Part model, mm, in its own coordinate system. A direction names the side the tool comes from. Round coordinates to 2 decimals unless told otherwise and drop trailing zeros. Loops run counter-clockwise (first coordinate to the right, second up) from the corner with the lowest first, then second, coordinate; pieces in that order, holes last.
from build123d import *

# Parameters (mm, degrees)
BOSS_EXTRUDE2_DEPTH                               = 5.08
CSK_FOR_8_FLAT_HEAD_MACHINE_SCREW_100_D           = 4.4958
CSK_FOR_8_FLAT_HEAD_MACHINE_SCREW_100_CSINK_D     = 8.89
CSK_FOR_8_FLAT_HEAD_MACHINE_SCREW_100_CSINK_ANGLE = 100
CUT_EXTRUDE1_DEPTH                                = 4.556
FILLET1_R                                         = 2.54
FILLET2_R                                         = 1.27


with BuildPart() as part:
    # Sketch4 → Boss-Extrude2 (new body, symmetric)
    with BuildSketch(Plane.XY):
        Polygon((0, 0), (4.445, 0), (4.445, 4.572), (8.001, 4.572), (8.001, -3.81), (0, -3.81), align=None)
    extrude(amount=BOSS_EXTRUDE2_DEPTH, both=True)

    # CSK for #8 Flat Head Machine Screw (100)2 (through all)
    with Locations(Plane(origin=(0, 0, 0), x_dir=(1, 0, 0), z_dir=(0, 1, 0))):
        with Locations((0, 0)):
            CounterSinkHole(CSK_FOR_8_FLAT_HEAD_MACHINE_SCREW_100_D / 2, CSK_FOR_8_FLAT_HEAD_MACHINE_SCREW_100_CSINK_D / 2, counter_sink_angle=CSK_FOR_8_FLAT_HEAD_MACHINE_SCREW_100_CSINK_ANGLE)

    # Sketch7 → Cut-Extrude1 (cut, through all)
    with BuildSketch(Plane.ZY.offset(-4.445)):
        with BuildLine():
            Line((-1.778, 2.032), (1.778, 2.032))
            ThreePointArc((1.778, 2.032), (2.794, 1.016), (1.778, 0))
            Line((1.778, 0), (-1.778, 0))
            ThreePointArc((-1.778, 0), (-2.794, 1.016), (-1.778, 2.032))
        make_face()
    extrude(amount=-CUT_EXTRUDE1_DEPTH, mode=Mode.SUBTRACT)

    # Fillet1
    fillet1_edges = [part.edges().sort_by_distance(p)[0] for p in [
        (6.223, 4.572, 5.08),
        (6.223, 4.572, -5.08),
    ]]
    fillet(fillet1_edges, radius=FILLET1_R)

    # Fillet2
    fillet2_edges = [part.edges().sort_by_distance(p)[0] for p in [
        (8.001, -0.889, 5.08),
        (8.001, 4.572, 0),
        (8.001, 3.828051224, 4.336051224),
        (8.001, 3.828051224, -4.336051224),
        (8.001, -0.889, -5.08),
    ]]
    fillet(fillet2_edges, radius=FILLET2_R)

    # Mirror2: part across plane


with BuildPart() as part_1:
    add(part.part)
    add(part.part.mirror(Plane(origin=(0, 0, 0), x_dir=(0, 0, 1), z_dir=(1, 0, 0))))


solid = part_1.part
1) Wall check: line 1 along Z through (x, y) = (0, -2.35); line 2 along X through (y, z) = (-2.4, 0); line 3 along Y through (x, z) = (-4.5, -1). Give the ranges that are in metal, low to high.
Values:
line 1: z = -5.08 to -2.25, 2.25 to 5.08
line 2: x = -8 to -2.25, 2.25 to 8
line 3: y = -3.81 to 0, 2.03 to 4.57
2) Slice it at D-D, the plane x = 0. Give the cut face in (y, z) (3 decimals).
Values:
outline: (-3.81, -5.08) - (0, -5.08) - (0, -4.445) - (-1.844, -2.248) - (-3.81, -2.248) - close; (-3.81, 2.248) - (-1.844, 2.248) - (0, 4.445) - (0, 5.08) - (-3.81, 5.08) - close
3) Mould opens along Y. For faces 4 (the face through (-7.619, -0.848, -4.718)), 5 (the face through (-6.198, 1.038, 2.794)), 6 (the face through (6, 4.572, 0)) say: released by +Y, released by -Y, zero draft, split by the parting line, or undercut.
Values:
face 4: zero draft
face 5: undercut
face 6: released by +Y
4) Slice it at A-A, the plane z = 0. Give the cut face in (x, y) (3 decimals).
Values:
outline: (-8.001, -3.81) - (-2.248, -3.81) - (-2.248, -1.844) - (-4.445, 0) - (-8.001, 0) - close; (-8.001, 2.032) - (-4.445, 2.032) - (-4.445, 4.572) - (-6.731, 4.572) arc R1.27 ccw to (-8.001, 3.302) - close; (2.248, -3.81) - (8.001, -3.81) - (8.001, 0) - (4.445, 0) - (2.248, -1.844) - close; (4.445, 2.032) - (8.001, 2.032) - (8.001, 3.302) arc R1.27 ccw to (6.731, 4.572) - (4.445, 4.572) - close
5) Tool access for faces 1 (the face through (5.604, 3.808, 4.356)), 2 (the face through (-4.445, 3, 0)), 3 (the face through (6, 2.032, 0)): list every direction of +Z, -Z, +X, -X, +Y, -Y with a clear straight run to the whole face (end or side of a thin tool).
Values:
face 1: +Z, +X, -X, +Y
face 2: +Z, -Z, +Y
face 3: +X, -X
6) Drop a flat-ended pin along its axis: pin 1 Ø1.5 at (x, y) = (-5.5, 3) entering from +Z. Give the stop position or say it passes through.
Values:
pin 1: stops at z = 5.07
7) Slice it at B-B, the plane x = -5.5. Give the cut face in (y, z).
Values:
outline: (-3.81, -5.08) - (2.03, -5.08) arc R2.54 ccw to (4.57, -2.54) - (4.57, 2.54) arc R2.54 ccw to (2.03, 5.08) - (-3.81, 5.08) - close; hole (0, -1.78) arc R1.02 ccw to (2.03, -1.78) - (2.03, 1.78) arc R1.02 ccw to (0, 1.78) - close
8) Slice it at C-C, the plane y = 1.25. Give the cut face in (x, z) (3 decimals).
Values:
outline: (-8.001, -3.81) arc R1.27 ccw to (-6.731, -5.08) - (-4.445, -5.08) - (-4.445, -2.767) - (-8.001, -2.767) - close; (-8.001, 2.767) - (-4.445, 2.767) - (-4.445, 5.08) - (-6.731, 5.08) arc R1.27 ccw to (-8.001, 3.81) - close; (4.445, -5.08) - (6.731, -5.08) arc R1.27 ccw to (8.001, -3.81) - (8.001, -2.767) - (4.445, -2.767) - close; (4.445, 2.767) - (8.001, 2.767) - (8.001, 3.81) arc R1.27 ccw to (6.731, 5.08) - (4.445, 5.08) - close
